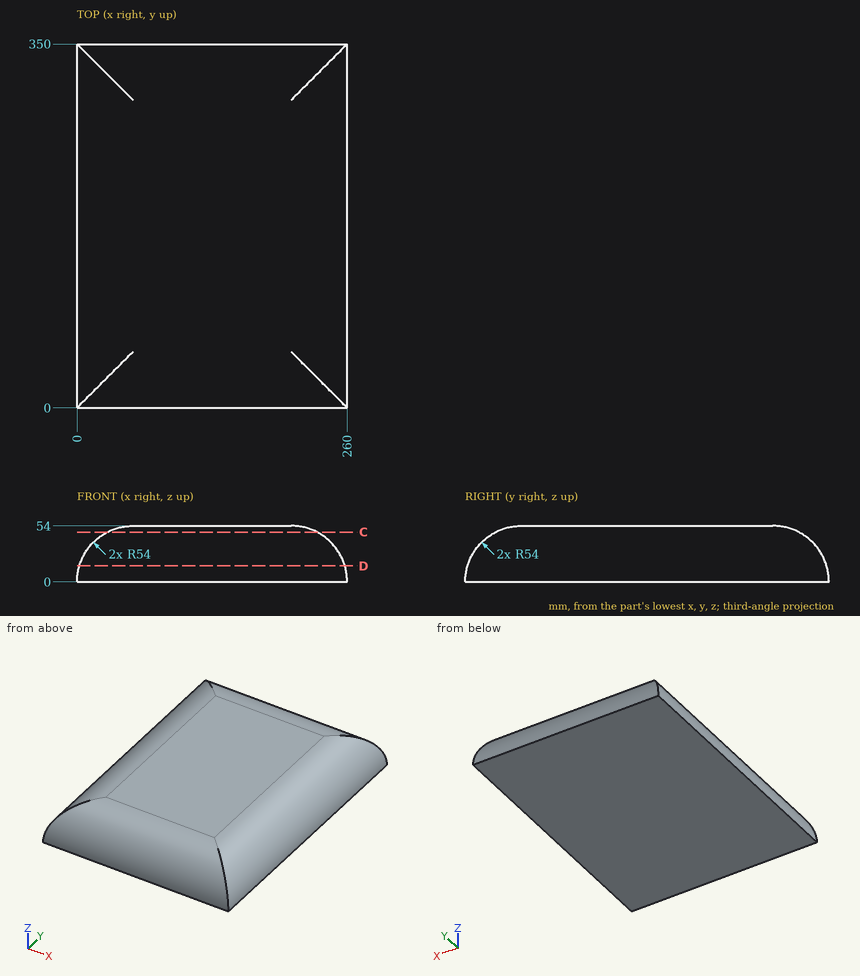
Here's the drawing with two shaded views (mm, measured from the low corner). I have some questions. Coordinates: 2 decimals unless noted, no trailing zeros. Order: outer loops, then holes, each group sorted by start corner. A loop starts at its lowest first (then second) coordinate and runs counter-clockwise, first axis right, second up. Notation, with made-up numbers: (-38.5, -9) - (9.5, -9) arc R18 cw to (9.5, 24) - close; hole circle Ø1 at (6.5, 80.5). An arc over 180 degrees is marked (long way). Answer in a Markdown table with one row per item. Add a question column.
(1) I need wall thicknesses on L1, parallel to X at y = 108, z = 41.5; L2, parallel to Z at x = 48, y = 123.5; L3, parallel to X at y = 80, z = 19.5. Which ranges of each line are inside material? Lowest first, please.
(2) If we section it at C-C, the plane z = 48: Please give me the cut outline in (x, y).
(3) If we section it at D-D, the plane z = 15.5: Please give me the cut outline in (x, y), then the cut area to 3 significant figures.
(4) Will these pins go through, and if not, where does the flat tip stop? pin 1 (4 mm diameter, centred on x = 156, z = 10, fed in from -Y); pin 2 (1.5 mm diameter, centred on x = 26.5, y = 70.5, fed in from -Z); pin 3 (12 mm diameter, centred on y = 131, z = 23.5, fed in from -X); pin 4 (2 mm diameter, centred on x = 62.5, y = 49.5, fed in from +Z).
Results are:
| question | item | result |
|---|---|---|
| 1 | L1 | x = 19.45 to 240.55 |
| 1 | L2 | z = 0 to 53.67 |
| 1 | L3 | x = 3.64 to 256.36 |
| 2 | outline | (29.26, 29.26) - (230.74, 29.26) - (230.74, 320.74) - (29.26, 320.74) - close |
| 3 | outline | (2.27, 2.27) - (257.73, 2.27) - (257.73, 347.73) - (2.27, 347.73) - close |
| 3 | area | 88,200 mm2 |
| 4 | pin 1 | stops at y = 0.6 |
| 4 | pin 2 | stops at z = 0 |
| 4 | pin 3 | stops at x = 2.91 |
| 4 | pin 4 | stops at z = 53.89 |
